Could you check a few things on this drawing? It's one solid part, dimensions in mm from its lowest x, y, z. Give positions to 0.01 mm unless a question says otherwise; leave off trailing zeros. Order: outer loops, then holes, each group sorted by start corner. A loop starts at its lowest first (then second) coordinate and runs counter-clockwise, first axis right, second up.
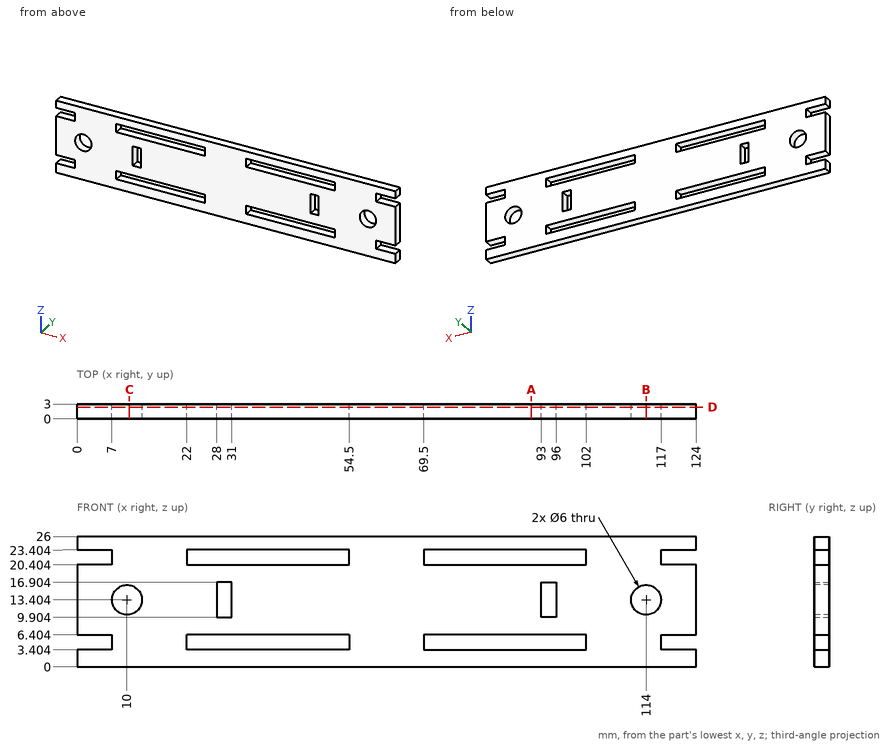
Item 1: Imagine slicing it at C-C on x = 10.5. List the corners of the cut face in (y, z) for me.
Findings:
outline: (0, 0) - (3, 0) - (3, 10.45) - (0, 10.45) - close; (0, 16.36) - (3, 16.36) - (3, 26) - (0, 26) - close
Item 2: For pin 1 (0.9 mm diameter, centred on y = 1, z = 21.5, fed in from +X), with a flat end and sliding along its axis, tell me the tip position at first contact or that it passes through.
Findings:
pin 1: stops at x = 117
Item 3: Please list where these lines run through material, in increasing order: line 1 along X through (y, z) = (2.7, 23.25); line 2 along Z through (x, y) = (91, 0.65); line 3 along Z through (x, y) = (93.5, 2.5).
Findings:
line 1: x = 7 to 22, 54.5 to 69.5, 102 to 117
line 2: z = 0 to 3.4, 6.4 to 20.4, 23.4 to 26
line 3: z = 0 to 3.4, 6.4 to 9.9, 16.9 to 20.4, 23.4 to 26
Item 4: Imagine slicing it at B-B on x = 114. List the corners of the cut face in (y, z) for me.
Findings:
outline: (0, 0) - (3, 0) - (3, 10.4) - (0, 10.4) - close; (0, 16.4) - (3, 16.4) - (3, 26) - (0, 26) - close
Item 5: Imagine slicing it at A-A on x = 91. List the corners of the cut face in (y, z) for me.
Findings:
outline: (0, 0) - (3, 0) - (3, 3.4) - (0, 3.4) - close; (0, 6.4) - (3, 6.4) - (3, 20.4) - (0, 20.4) - close; (0, 23.4) - (3, 23.4) - (3, 26) - (0, 26) - close
Item 6: Imagine slicing it at D-D on y = 2.35. Give the number of separate pieces and of enclosed holes in the cut face, then the cut area to 3 significant figures.
Findings:
separate pieces: 1
enclosed holes: 8
area: 2,650 mm2
